Geometry check sheet. Reference: the model listing, model coordinates, mm. Round coordinates to 2 decimals unless told otherwise and drop trailing zeros. Order: outer loops, then holes, each group sorted by start corner. A loop starts at its lowest first (then second) coordinate and runs counter-clockwise, first axis right, second up.
(1) Sectioned sample at B-B (y = 2). Give the number of separate pieces and of enclosed holes in the cut face, plus the area to 3 significant figures.
(2) Go/stop test with flat-tipped pins: pin 1 (9 mm diameter, centred on y = 1.5, z = -1, fed in from +X); pin 2 (1.5 mm diameter, centred on x = -2, y = -2.5, fed in from +Z); pin 3 (5 mm diameter, centred on x = -0.5, z = 6, fed in from -Y); pin 4 (1.5 mm diameter, centred on x = 3.5, y = -4.5, fed in from -Z). Record where each tip stops, or that it passes through.
(3) Material ranges on line 1 along X through (y, z) = (3.25, 3.5); line 2 along X through (y, z) = (1.25, 2.5); line 3 along Z through (x, y) = (1.75, 1.5), recorded low to high.
(4) Sectioned sample at A-A (x = -2.25). Record the boundary of the cut face in (y, z).
(5) Sectioned sample at D-D (y = 7.5). Record the boundary of the cut face in (x, z), plus the area to 3 significant figures.
(6) Sectioned sample at C-C (z = 5). Record the boundary of the cut face in (x, y).
from build123d import *
from build123d.topology import SkipClean

# Parameters (mm, degrees)
IZIM1_W               = 10.5
IZIM1_H               = 8
IZIM3_R               = 4
KES_EKSTR_ZYON1_DEPTH = 4
DI_1_PITCH            = 1


with BuildPart() as part:
    # Çizim1 → Döndür1 (revolve)
    with BuildSketch(Plane.XY, mode=Mode.PRIVATE) as d_nd_r1_sk:
        with Locations((-0.900163094, -2.913793103)):
            Rectangle(IZIM1_W, IZIM1_H)
    revolve(d_nd_r1_sk.sketch.rotate(Axis((-6.150163094, 1.086206897, 0), (1, 0, 0)), 270), axis=Axis((-6.150163094, 1.086206897, 0), (1, 0, 0)))

    # Çizim3 → Kes-Ekstrüzyon1 (cut)
    with BuildSketch(Plane(origin=(4.349836906, 0, 0), x_dir=(0, 0, -1), z_dir=(1, 0, 0))):
        with Locations((0, 1.086206897)):
            Circle(IZIM3_R)
    extrude(amount=-KES_EKSTR_ZYON1_DEPTH, mode=Mode.SUBTRACT)

    # Diş1: the profile of Diş Profili1 profile screwed along a right-hand helix of 4.5 turns, 8 arcs to a turn; built about Z, then put on its axis
    with SkipClean():  # the faces are left unmerged after this step: merging them gives an invalid solid
        di_1_z = Axis((0, 0, 0), (0, 0, 1))
        di_1_corners = [(3.9997, 0, -0.000173205), (4.541265875, 0, 0.312499999), (4.541265875, 0, 0.437499999), (3.9997, 0, 0.750173202)]
        with BuildLine(mode=Mode.PRIVATE) as di_1_profile:
            Line(di_1_corners[0], di_1_corners[1])
            Line(di_1_corners[1], di_1_corners[2])
            Line(di_1_corners[2], di_1_corners[3])
            Line(di_1_corners[3], di_1_corners[0])
        di_1_cap = Face(di_1_profile.wire())
        di_1_turn_angles = [0, 22.5, 45, 67.5, 90, 112.5, 135, 157.5, 180, 202.5, 225, 247.5, 270, 292.5, 315, 337.5, 360]
        di_1_turn_weights = [1, 0.9238795325112867, 1, 0.9238795325112867, 1, 0.9238795325112867, 1, 0.9238795325112867, 1, 0.9238795325112867, 1, 0.9238795325112867, 1, 0.9238795325112867, 1, 0.9238795325112867, 1]
        di_1_turn_rails = [Edge.make_bspline([Vector(p[0], p[1], 0).rotate(di_1_z, di_1_turn_angles[k]) / di_1_turn_weights[k] + Vector(0, 0, p[2] + DI_1_PITCH * di_1_turn_angles[k] / 360) for k in range(17)], [0, 0, 0, 1, 1, 2, 2, 3, 3, 4, 4, 5, 5, 6, 6, 7, 7, 8, 8, 8], 2, di_1_turn_weights) for p in di_1_corners]
        di_1_turn_sides = [Face.make_surface_from_curves(di_1_turn_rails[p[0]], di_1_turn_rails[p[1]]) for p in [(0, 1), (1, 2), (2, 3), (3, 0)]]
        di_1_last_angles = [1440, 1462.5, 1485, 1507.5, 1530, 1552.5, 1575, 1597.5, 1620]
        di_1_last_weights = [1, 0.9238795325112867, 1, 0.9238795325112867, 1, 0.9238795325112867, 1, 0.9238795325112867, 1]
        di_1_last_rails = [Edge.make_bspline([Vector(p[0], p[1], 0).rotate(di_1_z, di_1_last_angles[k]) / di_1_last_weights[k] + Vector(0, 0, p[2] + DI_1_PITCH * di_1_last_angles[k] / 360) for k in range(9)], [0, 0, 0, 1, 1, 2, 2, 3, 3, 4, 4, 4], 2, di_1_last_weights) for p in di_1_corners]
        di_1_last_sides = [Face.make_surface_from_curves(di_1_last_rails[p[0]], di_1_last_rails[p[1]]) for p in [(0, 1), (1, 2), (2, 3), (3, 0)]]
        di_1 = Plane(origin=(4.349836906, 1.086206897, 0), x_dir=(0, 0, 1), z_dir=(-1, 0, 0)) * Solid(Shell([*[p.moved(Location((0, 0, DI_1_PITCH * i))) for i in range(4) for p in di_1_turn_sides], *di_1_last_sides, di_1_cap, di_1_cap.rotate(di_1_z, 1620).moved(Location((0, 0, DI_1_PITCH * 1620 / 360)))]))
        add(di_1, mode=Mode.SUBTRACT)


solid = part.part
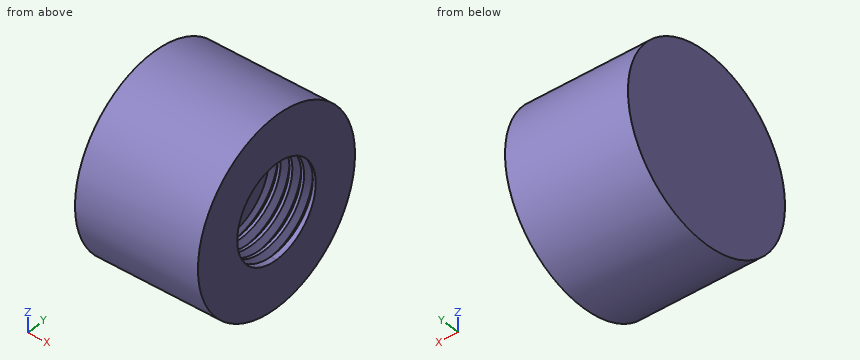
Answer below:
1. separate pieces: 1
1. enclosed holes: 2
1. area: 133 mm2
2. pin 1: stops at x = 4.35
2. pin 2: stops at z = 7.48
2. pin 3: stops at y = -6.11
2. pin 4: stops at z = -6.37
3. line 1: x = -6.15 to -0.42, 0.19 to 0.58, 1.19 to 1.58, 2.19 to 2.58, 3.19 to 3.58, 4.19 to 4.35
3. line 2: x = -6.15 to 0.35
3. line 3: z = -7.99 to -4.18, 4.27 to 7.99
4. outline: circle Ø16 at (1.09, 0)
5. outline: (-6.15, -4.78) - (4.35, -4.78) - (4.35, 4.78) - (-6.15, 4.78) - close
5. area: 100 mm2
6. outline: (-6.15, -5.16) - (4.35, -5.16) - (4.35, 7.33) - (-6.15, 7.33) - close
